from build123d import *

# Parameters (mm, degrees)
BOSS_EXTRUDE1_DEPTH = 5.7


with BuildPart() as part:
    # Sketch1 → Boss-Extrude1 (new body)
    with BuildSketch(Plane(origin=(0, 0, 0), x_dir=(1, 0, 0), z_dir=(0, 1, 0))):
        with BuildLine():
            Line((0, 0), (0, 301.474))
            add(Edge.make_bspline(
                [(0, 301.474), (1.947152909, 355.934632045), (-16.543745931, 407.327520261)],
                knots=[0, 0, 0, 1, 1, 1], degree=2))
            Line((-16.543745931, 407.327520261), (-12.38816914, 411.710423204))
            add(Edge.make_bspline(
                [(5.7, 331.474), (2.429624829, 372.720008317), (-12.38816914, 411.710423204)],
                knots=[0, 0, 0, 1, 1, 1], degree=2))
            Line((5.7, 331.474), (5.7, 0))
            Line((5.7, 0), (5.7, -0.427567417))
            Line((5.7, -0.427567417), (0, 0))
        make_face()
    extrude(amount=BOSS_EXTRUDE1_DEPTH)


solid = part.part
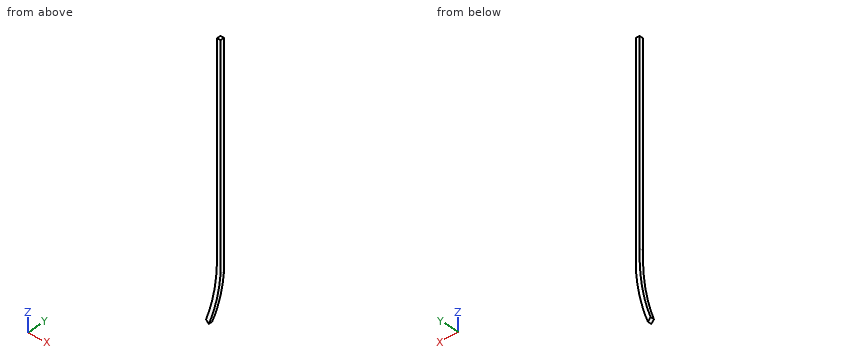
Could you check a few things on this model? Use its own coordinates, in mm. Give positions to 0.01 mm unless a question says otherwise; leave off trailing zeros. Write each loop counter-clockwise with the first axis right and the second up, starting at its lowest first coordinate (ties: lowest second). Pieces come first, ordered by that corner, then holes. Notation, with made-up numbers: (10.5, 76) -> (41.5, 76) arc R15 ccw to (41.5, 81) -> close; hole circle Ø3 at (-29.5, 30.25). An arc over 180 degrees is marked (long way). Write each question's results on one line, items separated by ' | '. Start each with the question number.
Q1. I need wall thicknesses on probe 1 along X at (y, z) = (4, -265.5); probe 2 along X at (y, z) = (0.45, -367). Which ranges of each line are inside material? Lowest first, please.
Q2. I'm going to push flat-ended pins straight in: pin 1 Ø3 at (y, z) = (2, -167) entering from -X; pin 2 Ø2 at (x, y) = (0.5, 4.5) entering from +Z; pin 3 Ø1 at (x, z) = (-1.5, -264.5) entering from +Y. Where does each tip first touch, or does it pass through?
Q3. Suppose I cut it at A-A, the plane z = -265.5. List the corners of the cut face in (x, y) for me.
Outcome:
1) probe 1: 0 to 5.7 | probe 2: -5.27 to 0.66
2) pin 1: x = 0 | pin 2: z = 0.11 | pin 3: through
3) outline: (0, 0) -> (5.7, 0) -> (5.7, 5.7) -> (0, 5.7) -> close
